The listing builds one solid part. Answer for the finished solid, in the listing's coordinates (mm). A direction names the side the tool comes from. Coordinates: 2 decimals unless noted, no trailing zeros. Write each loop counter-clockwise with the first axis right and the second up, starting at its lowest first coordinate (ties: lowest second). Pieces come first, ordered by that corner, then holes.
from build123d import *

# Parameters (mm, degrees)
BOSS_EXTRUDE1_DEPTH = 36.5
BOSS_EXTRUDE2_DEPTH = 6
BOSS_EXTRUDE3_DEPTH = 15
BOSS_EXTRUDE4_DEPTH = 18
CUT_EXTRUDE2_DEPTH  = 25
SKETCH5_W           = 21
SKETCH5_H           = 37.8
CUT_EXTRUDE1_DEPTH  = 32
FILLET1_R           = 10
CUT_EXTRUDE3_DEPTH  = 18
SKETCH9_W           = 81.549954628
SKETCH9_H           = 20
CUT_EXTRUDE4_DEPTH  = 18
SKETCH10_W          = 7.5
SKETCH10_H          = 36.5
CUT_EXTRUDE6_DEPTH  = 106.049226723


with BuildPart() as part:
    # Sketch1 → Boss-Extrude1 (new body)
    with BuildSketch(Plane(origin=(0, 0, 0), x_dir=(1, 0, 0), z_dir=(0, 1, 0))):
        with BuildLine():
            Line((-62.5, -34.2), (-62.5, -35.745629103))
            ThreePointArc((-62.5, -35.745629103), (0, -72), (62.5, -35.745629103))
            Line((62.5, -35.745629103), (62.5, -34.2))
            Line((62.5, -34.2), (-62.5, -34.2))
        make_face()
    extrude(amount=-BOSS_EXTRUDE1_DEPTH)

    # Sketch2 → Boss-Extrude2 (add)
    with BuildSketch(Plane.XZ.offset(36.5)):
        with BuildLine():
            ThreePointArc((39.5, 60.197591314), (0, 72), (-39.5, 60.197591314))
            Line((-39.5, 60.197591314), (-39.5, 34.2))
            Line((-39.5, 34.2), (39.5, 34.2))
            Line((39.5, 34.2), (39.5, 60.197591314))
        make_face()
    extrude(amount=BOSS_EXTRUDE2_DEPTH)

    # Sketch3 → Boss-Extrude3 (add)
    with BuildSketch(Plane.XZ.offset(42.5)):
        with BuildLine():
            Line((-32, 64.498061986), (-32, 34.2))
            Line((-32, 34.2), (32, 34.2))
            Line((32, 34.2), (32, 64.498061986))
            ThreePointArc((32, 64.498061986), (0, 72), (-32, 64.498061986))
        make_face()
    extrude(amount=BOSS_EXTRUDE3_DEPTH)

    # Sketch4 → Boss-Extrude4 (add)
    with BuildSketch(Plane.XZ.offset(57.5)):
        with BuildLine():
            Line((-24.5, 34.2), (-24.5, 67.703397256))
            ThreePointArc((-24.5, 67.703397256), (0, 72), (24.5, 67.703397256))
            Line((24.5, 67.703397256), (24.5, 34.2))
            Line((24.5, 34.2), (-24.5, 34.2))
        make_face()
    extrude(amount=BOSS_EXTRUDE4_DEPTH)

    # Sketch7 → Cut-Extrude2 (cut)
    with BuildSketch(Plane(origin=(0, 0, 34.2), x_dir=(-1, 0, 0), z_dir=(0, 0, -1))):
        with BuildLine():
            Line((-32.5, -53.5), (-32.5, -86))
            Line((-32.5, -86), (32.5, -86))
            Line((32.5, -86), (32.5, -53.5))
            ThreePointArc((32.5, -53.5), (0, -21), (-32.5, -53.5))
        make_face()
    extrude(amount=-CUT_EXTRUDE2_DEPTH, mode=Mode.SUBTRACT)

    # Sketch5 → Cut-Extrude1 (cut)
    with BuildSketch(Plane.XZ.offset(75.5)):
        with Locations((0, 53.1)):
            Rectangle(SKETCH5_W, SKETCH5_H)
    extrude(amount=-CUT_EXTRUDE1_DEPTH, mode=Mode.SUBTRACT)

    # Fillet1
    fillet1_edges = [part.edges().sort_by_distance(p)[0] for p in [
        (-10.5, -43.5, 65.215130212),
        (10.5, -43.5, 65.215130212),
    ]]
    fillet(fillet1_edges, radius=FILLET1_R)

    # Sketch8 → Cut-Extrude3 (cut)
    with BuildSketch(Plane(origin=(0, 0, 34.2), x_dir=(-1, 0, 0), z_dir=(0, 0, -1))):
        with BuildLine():
            Line((-27, -2), (27, -2))
            ThreePointArc((27, -2), (47, -22), (27, -42))
            Line((27, -42), (-27, -42))
            ThreePointArc((-27, -42), (-47, -22), (-27, -2))
        make_face()
    extrude(amount=-CUT_EXTRUDE3_DEPTH, mode=Mode.SUBTRACT)

    # Sketch9 → Cut-Extrude4 (cut)
    with BuildSketch(Plane(origin=(0, 0, 34.2), x_dir=(-1, 0, 0), z_dir=(0, 0, -1))):
        with Locations((0, -46.5)):
            Rectangle(SKETCH9_W, SKETCH9_H)
    extrude(amount=-CUT_EXTRUDE4_DEPTH, mode=Mode.SUBTRACT)

    # Sketch10 → Cut-Extrude6 (cut, through all)
    with BuildSketch(Plane(origin=(0, 0, 34.2), x_dir=(-1, 0, 0), z_dir=(0, 0, -1))):
        with Locations((-58.75, -18.25)):
            Rectangle(SKETCH10_W, SKETCH10_H)
    extrude(amount=-CUT_EXTRUDE6_DEPTH, mode=Mode.SUBTRACT)


solid = part.part
1. Section D-D on y = -23.5 is taken. Give the vertices of the cut face in (x, z), then the cut area to 3 significant figures.
Results found:
outline: (-62.5, 34.2) - (-46.94, 34.2) - (-46.94, 52.2) - (-12.5, 52.2) - (-12.5, 59.2) - (12.5, 59.2) - (12.5, 52.2) - (46.94, 52.2) - (46.94, 34.2) - (55, 34.2) - (55, 46.47) arc R72 ccw to (-62.5, 35.75) - close
area: 1,490 mm2
2. Section C-C on z = 40 is taken. Give the vertices of the cut face in (x, y).
Results found:
outline: (-59.87, -36.5) - (-40.77, -36.5) arc R20 cw to (-27, -2) - (27, -2) arc R20 cw to (40.77, -36.5) - (55, -36.5) - (55, 0) - (-59.87, 0) - close
3. Flat-ended cylindrical pins translate along their axes: P1, Ø17, axis at x = 49, z = 51.5, coming from the -Y side; P2, Ø9.5, axis at y = -64.5, z = 66.5, coming from the -X side; P3, Ø13.5, axis at y = -53, z = 57, coming from the +X side. Find the tip coordinate at first contact, or state that the pin passes through.
Results found:
P1: stops at y = -36.5
P2: stops at x = -24.5
P3: stops at x = 32
4. Find the intervals of material crossed by L1, parallel to X at y = -11.5, z = 42.5; L2, parallel to X at y = -8, z = 64.5; L3, parallel to Y at x = -42.5, z = 41, in increasing order.
Results found:
L1: x = -58.12 to -44.02, 44.02 to 55
L2: x = -32 to 32
L3: y = -36.5 to -34.64, -9.36 to 0
5. A tool of negligible diameter and unlimited length cuts with its end or side. For faces 1 (the flat face through (-10.5, -65, 65)), 2 (the flat face through (1, -19, 52.2)), 3 (the flat face through (0, -42, 59.2)), 4 (the flat face through (-32, -48, 60)), 5 (the flat face through (39.5, -39, 56)), from which of +Z, -Z, +X, -X, +Y, -Y can it reach the whole face along a straight path? Write none if from no direction.
Results found:
face 1: +Z, -Z, -Y
face 2: -Z
face 3: -Z, -Y
face 4: +Z, -Z, -X, -Y
face 5: +Z, -Z, +X, -Y
6. For a pull along X with two mould halves and no side action, classify faces 6 (the flat face through (32, -48, 60)), 7 (the cylindrical face through (-45.45, -14.28, 43.07)), 8 (the cylindrical face through (45.695, -14.895, 43.074)), 9 (the flat face through (47, -36.5, 44)) as pulls with the +X half, pulls with the -X half, needs draft (parallel to the pull), parting line crosses it, or undercut.
Results found:
face 6: pulls with the +X half
face 7: undercut
face 8: undercut
face 9: needs draft
7. Section A-A on y = -62 is taken. Give the vertices of the cut face in (x, z).
Results found:
outline: (-24.5, 59.2) - (-10.5, 59.2) - (-10.5, 71.23) arc R72 ccw to (-24.5, 67.7) - close; (10.5, 59.2) - (24.5, 59.2) - (24.5, 67.7) arc R72 ccw to (10.5, 71.23) - close
8. Section B-B on y = -6 is taken. Give the vertices of the cut face in (x, z).
Results found:
outline: (-62.5, 34.2) - (-39, 34.2) - (-39, 52.2) - (39, 52.2) - (39, 34.2) - (55, 34.2) - (55, 46.47) arc R72 ccw to (-62.5, 35.75) - close
